Geometry: final body of the model. Coordinates: model frame, mm. Face numbers are marked on the shaded views. A direction names the side the tool comes from. Round coordinates to 2 decimals unless told otherwise and drop trailing zeros. Order: outer loops, then holes, each group sorted by start corner. A loop starts at its lowest first (then second) coordinate and runs counter-clockwise, first axis right, second up. Notation, with made-up numbers: M 15,32 L 74,32 A26 cw 74,54 Z; hole C 45.5,-7.5 d11. An arc over 180 degrees is marked long. Put each result on its own line as item: value. Start each with the question number.
1) Access query for the marked faces 1, 2 and 3. Directions: +Z, -Z, +X, -X, +Y, -Y. A direction counts if a zero-diameter tool reaches every point of the face in a straight line with its end or side. Return the directions, or none.
2) Draft query along X for the marked faces 4, 5 and 6. Return one class per face: pulls with the +X half, pulls with the -X half, needs draft (parallel to the pull), parting line crosses it, or undercut.
3) Material intervals for probe 1 along Y at (x, z) = (0.8, 0.6); probe 2 along Y at (x, z) = (0.3, -1.75); probe 3 along X at (y, z) = (-7.75, -0.7), sorted ascending. Write a range as [from, to].
4) Section A-A, the plane z = 0. Return loops of the section in (x, y).
5) First-contact query: P1, Ø1, axis at y = -6, z = -0.5, coming from the -X side; P2, Ø1.5, axis at y = -5.5, z = -2, coming from the +X side; P3, Ø1.5, axis at x = 0, z = 1.5, coming from the -Y side. Flat tips, straight axial feed; report the tip coordinate or a pass-through.
6) Section B-B, the plane y = -8.25. Return loops of the section in (x, z), then the cut area to 3 significant figures.
from build123d import *

# Parameters (mm, degrees)
CHAMFER1_SIZE      = 0.25
FILLET1_R          = 0.2
CUT_EXTRUDE1_DEPTH = 2
FILLET2_R          = 0.1


with BuildPart() as part:
    # Sketch1 → Revolve1 (revolve)
    with BuildSketch(Plane.XY):
        Polygon((0, -11), (-1.5, -11), (-1.5, -3), (-2.75, -3), (-2.75, 0), (0, 0), align=None)
    revolve(axis=Axis((0, 0, 0), (0, -1, 0)))

    # Chamfer1
    chamfer1_edges = [part.edges().sort_by_distance(p)[0] for p in [
        (1.5, -3, 0),
        (1.5, -11, 0),
    ]]
    chamfer(chamfer1_edges, length=CHAMFER1_SIZE)

    # Fillet1
    fillet1_edges = [part.edges().sort_by_distance(p)[0] for p in [
        (2.75, 0, 0),
    ]]
    fillet(fillet1_edges, radius=FILLET1_R)

    # Sketch2 → Cut-Extrude1 (cut)
    with BuildSketch(Plane(origin=(0, 0, 0), x_dir=(1, 0, 0), z_dir=(0, 1, 0))):
        Polygon((0, 1.443375673), (-1.25, 0.721687836), (-1.25, -0.721687836), (0, -1.443375673), (1.25, -0.721687836), (1.25, 0.721687836), align=None)
    extrude(amount=-CUT_EXTRUDE1_DEPTH, mode=Mode.SUBTRACT)

    # Fillet2
    fillet2_edges = [part.edges().sort_by_distance(p)[0] for p in [
        (0.625, -2, -1.082531755),
        (1.25, -2, 0),
        (0.625, -2, 1.082531755),
        (-0.625, -2, 1.082531755),
        (-1.25, -2, 0),
        (-0.625, -2, -1.082531755),
        (0.625, 0, -1.082531755),
        (-0.625, 0, -1.082531755),
        (-1.25, 0, 0),
        (-0.625, 0, 1.082531755),
        (0.625, 0, 1.082531755),
        (1.25, 0, 0),
    ]]
    fillet(fillet2_edges, radius=FILLET2_R)


solid = part.part
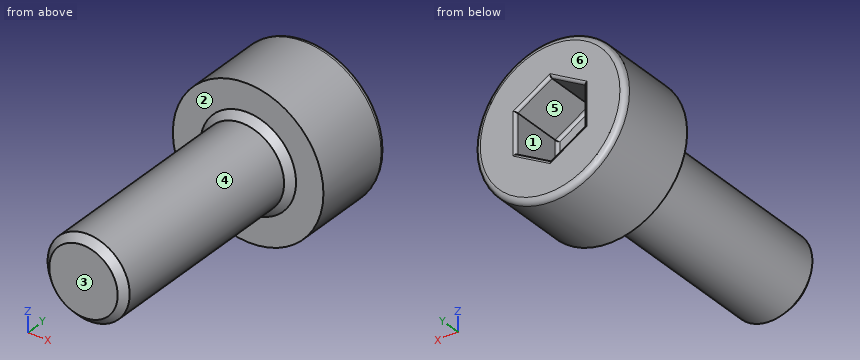
Result sheet:
1. face 1: +Y
1. face 2: -Y
1. face 3: +Z, -Z, +X, -X, -Y
2. face 4: parting line crosses it
2. face 5: undercut
2. face 6: needs draft
3. probe 1: y = [-11, -2]
3. probe 2: y = [-3, 0]
3. probe 3: x = [-1.33, 1.33]
4. outline: M -2.75,-3 L -1.75,-3 L -1.5,-3.25 L -1.5,-10.75 L -1.25,-11 L 1.25,-11 L 1.5,-10.75 L 1.5,-3.25 L 1.75,-3 L 2.75,-3 L 2.75,-0.2 A0.2 ccw 2.55,0 L 1.35,0 A0.1 ccw 1.25,-0.1 L 1.25,-1.9 A0.1 cw 1.15,-2 L -1.15,-2 A0.1 cw -1.25,-1.9 L -1.25,-0.1 A0.1 ccw -1.35,0 L -2.55,0 A0.2 ccw -2.75,-0.2 Z
5. P1: stops at x = -1.5
5. P2: stops at x = 0.83
5. P3: stops at y = -11
6. outline: C 0,0 d3
6. area: 7.07 mm2
